Verification items for the finished model (mm, model axes). Face numbers are marked on the shaded views. A direction names the side the tool comes from. Give positions to 0.01 mm unless a question says otherwise; leave off trailing zeros. Loops run counter-clockwise (first coordinate to the right, second up) from the corner with the lowest first, then second, coordinate; pieces in that order, holes last. Notation, with made-up numbers: M -19.75,7.5 L 33.25,7.5 A9 cw 33.25,13.5 Z; hole C 70.5,18 d10. An arc over 180 degrees is marked long. Write each question's results on one line, items separated by ' | '. Start each with the question number.
```python
from build123d import *

# Parameters (mm, degrees)
F1_DEPTH  = 12.7
F3_DEPTH  = 38.1
F4_W      = 19.05
F4_H      = 12.7
F5_DEPTH  = 50.801
F7_START  = -25.4
F6_W      = 25.4
F6_H      = 12.7
F7_DEPTH  = 72.90484
F9_DEPTH  = 25.401
F11_DEPTH = 25.401


with BuildPart() as f1:
    # F0 (on Top) → F1 (new body, symmetric)
    with BuildSketch(Plane.XY):
        Polygon((0, 15.875), (0, 0), (101.6, 0), (101.6, 15.875), (82.55, 15.875), (82.55, 34.925), (101.6, 34.925), (101.6, 50.8), (0, 50.8), (0, 34.925), (19.05, 34.925), (19.05, 15.875), align=None)
    extrude(amount=F1_DEPTH, both=True)

    # F2 (on face) → F3 (join)
    with BuildSketch(Plane.XY.offset(12.7)):
        Polygon((76.2, 50.8), (25.4, 50.8), (50.8, 0), align=None)
    extrude(amount=F3_DEPTH)

    # F4 (on face) → F5 (cut, through all)
    with BuildSketch(Plane.XZ):
        with Locations((9.525, -6.35)):
            Rectangle(F4_W, F4_H)
        with BuildLine():
            Line((31.75, -12.7), (69.85, -12.7))
            Line((69.85, -12.7), (69.85, -6.35))
            ThreePointArc((69.85, -6.35), (67.9901280605, -1.8598719395), (63.5, 0))
            Line((63.5, 0), (38.1, 0))
            ThreePointArc((38.1, 0), (33.6098719395, -1.8598719395), (31.75, -6.35))
            Line((31.75, -6.35), (31.75, -12.7))
        make_face()
        with Locations((92.075, -6.35)):
            Rectangle(F4_W, F4_H)
    extrude(amount=-F5_DEPTH, mode=Mode.SUBTRACT)

    # F6 (on face) → F7 (cut)
    with BuildSketch(Plane(origin=(0, 50.8, 0), x_dir=(-1, 0, 0), z_dir=(0, 1, 0)).offset(F7_START)):
        with Locations((-50.8, 31.75)):
            Rectangle(F6_W, F6_H)
    extrude(amount=-F7_DEPTH, mode=Mode.SUBTRACT)

    # F8 (on face) → F9 (cut, through all)
    with BuildSketch(Plane.XY.offset(12.7)):
        with BuildLine():
            Line((0, 50.8), (0, 42.8625))
            ThreePointArc((0, 42.8625), (1.8247273895, 47.9848874708), (6.4769983292, 50.8))
            Line((6.4769983292, 50.8), (0, 50.8))
        make_face()
        with BuildLine():
            ThreePointArc((6.35, 0), (2.2840161092, 1.4262701365), (0, 5.08))
            Line((0, 5.08), (0, 0))
            Line((0, 0), (6.35, 0))
        make_face()
    extrude(amount=-F9_DEPTH, mode=Mode.SUBTRACT)

    # F10 (on face) → F11 (cut, through all)
    with BuildSketch(Plane.XY.offset(12.7)):
        with BuildLine():
            Line((101.6, 50.8), (95.25, 50.8))
            ThreePointArc((95.25, 50.8), (99.3159838908, 49.3737298635), (101.6, 45.72))
            Line((101.6, 45.72), (101.6, 50.8))
        make_face()
        with BuildLine():
            ThreePointArc((101.6, 5.08), (99.3159838908, 1.4262701365), (95.25, 0))
            Line((95.25, 0), (101.6, 0))
            Line((101.6, 0), (101.6, 5.08))
        make_face()
    extrude(amount=-F11_DEPTH, mode=Mode.SUBTRACT)


solid = f1.part
```
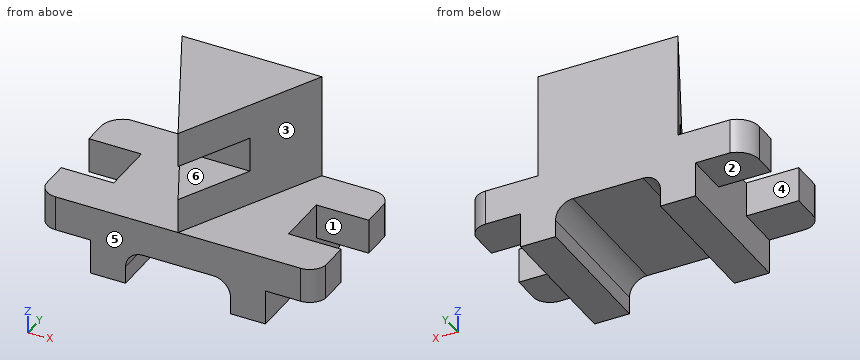
1. Release check for a two-part mould opening along Y. For the marked faces 4, 5 and 6 record: released by +Y, released by -Y, zero draft, split by the parting line, or undercut.
2. Depth check by flat-ended pin: pin 1 Ø5 at (x, y) = (36, 7) entering from +Z; pin 2 Ø3 at (y, z) = (26.5, -8.5) entering from -X; pin 3 Ø12.5 at (x, y) = (12, 44) entering from -Z. Enter the tip coordinate at first touch or a pass-through.
3. Section check B-B, the plane x = 13. Record the boundary of the cut face in (y, z) (3 decimals).
4. Set-up check for the marked faces 1, 2 and 3: record each of +Z, -Z, +X, -X, +Y, -Y from which the full face is reachable in a straight line by a thin tool's end or side.
5. Thickness scan on probe 1 along Y at (x, z) = (95, 0.5) (3 decimals); probe 2 along Z at (x, y) = (31.5, 36); probe 3 along Z at (x, y) = (13, 2). Record the ranges inside material, lowest first.
6. Section check A-A, the plane y = 12. Record the boundary of the cut face in (x, z).
7. Section check D-D, the plane y = 40. Record the boundary of the cut face in (x, z).
8. Section check C-C, the plane z = -3.5. Record the boundary of the cut face in (x, y), plus the area to 3 significant figures.
Filled sheet:
1) face 4: undercut | face 5: released by -Y | face 6: zero draft
2) pin 1: z = 12.7 | pin 2: x = 19.05 | pin 3: z = 0
3) outline: M 0,0 L 15.875,0 L 15.875,12.7 L 0,12.7 Z; M 34.925,0 L 50.8,0 L 50.8,12.7 L 34.925,12.7 Z
4) face 1: +Z, -Z, +X | face 2: -Z, -X, +Y, -Y | face 3: +Z, +X, -Y
5) probe 1: 0 to 15.875, 34.925 to 50.8 | probe 2: -12.7 to 12.7 | probe 3: 0 to 12.7
6) outline: M 0,0 L 19.05,0 L 19.05,-12.7 L 31.75,-12.7 L 31.75,-6.35 A6.35 cw 38.1,0 L 63.5,0 A6.35 cw 69.85,-6.35 L 69.85,-12.7 L 82.55,-12.7 L 82.55,0 L 101.6,0 L 101.6,12.7 L 56.8,12.7 L 56.8,25.4 L 44.8,25.4 L 44.8,12.7 L 0,12.7 Z; M 44.8,38.1 L 56.8,38.1 L 56.8,50.8 L 44.8,50.8 Z
7) outline: M 0,0 L 19.05,0 L 19.05,-12.7 L 31.75,-12.7 L 31.75,-6.35 A6.35 cw 38.1,0 L 63.5,0 A6.35 cw 69.85,-6.35 L 69.85,-12.7 L 82.55,-12.7 L 82.55,0 L 101.6,0 L 101.6,12.7 L 70.8,12.7 L 70.8,50.8 L 30.8,50.8 L 30.8,12.7 L 0,12.7 Z
8) outline: M 19.05,0 L 32.43,0 L 32.43,50.8 L 19.05,50.8 Z; M 69.17,0 L 82.55,0 L 82.55,50.8 L 69.17,50.8 Z | area: 1,360 mm2
